Print and shaded views of the part. All mm, measured from the part's lowest x, y and z. Give positions to 0.01 mm unless a question says otherwise; leave off trailing zeros. Loops run counter-clockwise (first coordinate to the right, second up) from the corner with the lowest first, then second, coordinate; pieces in that order, holes last.
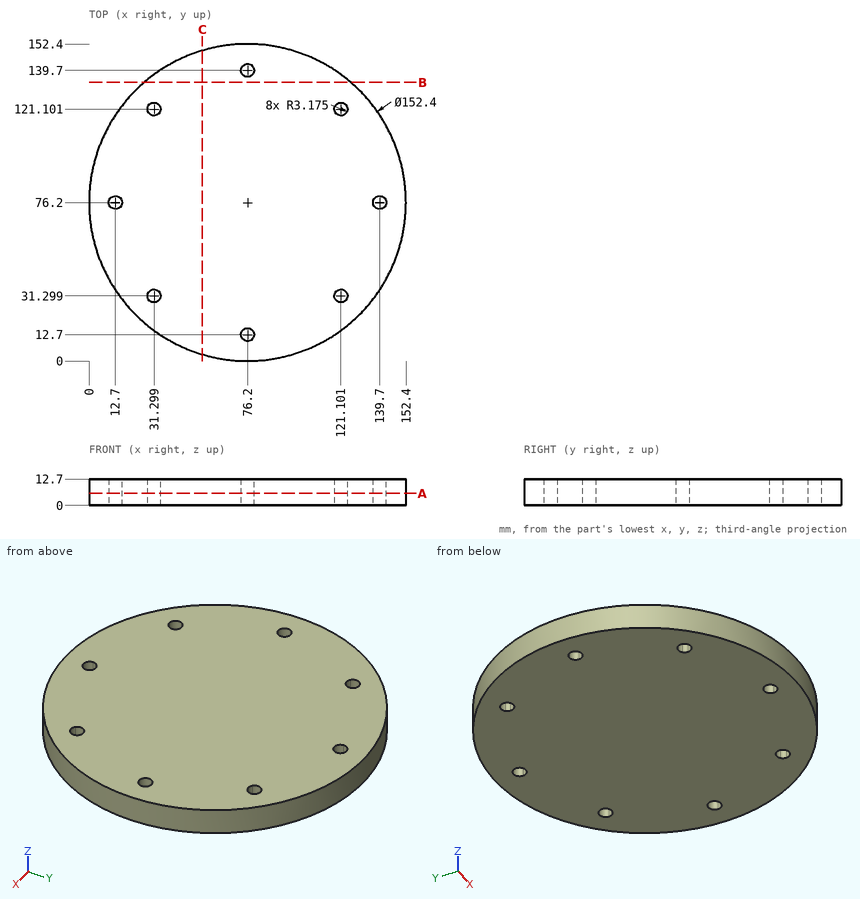
1. Probe line 1 along X through (y, z) = (33.5, 6.5); line 2 along Y through (x, z) = (14, 2.75) (1 decimal); line 3 along X through (y, z) = (74, 3). List the from-to ranges inside material, lowest first.
Responses:
line 1: x = 13.09 to 29.01, 33.59 to 118.81, 123.39 to 139.31
line 2: y = 32.2 to 73.3, 79.1 to 120.2
line 3: x = 0.03 to 10.41, 14.99 to 137.41, 141.99 to 152.37
2. Saw through at C-C, the plane x = 54.5. List the corners of the cut face in (y, z) (1 decimal), and give its area (3 significant figures).
Responses:
outline: (3.2, 0) - (149.2, 0) - (149.2, 12.7) - (3.2, 12.7) - close
area: 1,860 mm2
3. Drop flat-ended pins along their axis: pin 1 (4 mm diameter, centred on x = 103, z = 7.5, fed in from +Y); pin 2 (2 mm diameter, centred on y = 71, z = 4, fed in from +X); pin 3 (1.5 mm diameter, centred on x = 62.5, z = 5, fed in from +Y). Give the stop position or say it passes through.
Responses:
pin 1: stops at y = 148.25
pin 2: stops at x = 152.28
pin 3: stops at y = 151.29
4. Saw through at A-A, the plane z = 5.75. Count the separate pieces of the cut face and the enclosed holes in it, and give its area (3 significant figures).
Responses:
separate pieces: 1
enclosed holes: 8
area: 18,000 mm2
5. Saw through at B-B, the plane y = 134. List the corners of the cut face in (x, z) (1 decimal).
Responses:
outline: (26.5, 0) - (125.9, 0) - (125.9, 12.7) - (26.5, 12.7) - close
